```python
from build123d import *

# Parameters (mm, degrees)
M12X1_5_1_D              = 10.5
PATTERN_CIRCULAR_1_COUNT = 8
CHAMFER_1_SIZE           = 8
CHAMFER_2_SIZE           = 2


with BuildPart() as part:
    # 草圖1 → 旋轉1 (revolve)
    with BuildSketch(Plane.XY, mode=Mode.PRIVATE) as revolve_1_sk:
        Polygon((50, 0), (85, 0), (85, 30), (60, 30), (60, 540), (85, 540), (85, 570), (50, 570), align=None)
    revolve(revolve_1_sk.sketch.rotate(Axis((0, -1001.13524313, 0), (0, 1, 0)), 90), axis=Axis((0, -1001.13524313, 0), (0, 1, 0)))

    # 草圖2 → 除料-旋轉1 (revolve, cut)
    with BuildSketch(Plane.XY, mode=Mode.PRIVATE) as cut_revolve_1_sk:
        with BuildLine():
            Line((60, 540), (60, 532))
            ThreePointArc((60, 532), (58, 536), (60, 540))
        make_face()
        with BuildLine():
            Line((60, 38), (60, 30))
            ThreePointArc((60, 30), (58, 34), (60, 38))
        make_face()
    revolve(cut_revolve_1_sk.sketch.rotate(Axis((0, -1001.13524313, 0), (0, -1, 0)), 90), axis=Axis((0, -1001.13524313, 0), (0, -1, 0)), mode=Mode.SUBTRACT)

    # M12x1.5 螺紋孔1 (through all)
    with Locations(Plane.XZ):
        with Locations((-64.671567276, 26.787840266)):
            m12x1_5_1 = Hole(M12X1_5_1_D / 2)

    # 環狀複製排列1: M12x1.5 螺紋孔1 ×8 about axis
    pattern_circular_1_axis = Axis((0, 0, 0), (0, 1, 0))
    for i in range(1, PATTERN_CIRCULAR_1_COUNT):
        add(m12x1_5_1.rotate(pattern_circular_1_axis, i * 360 / PATTERN_CIRCULAR_1_COUNT), mode=Mode.SUBTRACT)

    # 導角1
    chamfer_1_edges = [part.edges().sort_by_distance(p)[0] for p in [
        (0, 540, 85),
        (0, 30, 85),
    ]]
    chamfer(chamfer_1_edges, length=CHAMFER_1_SIZE)

    # 導角2
    chamfer_2_edges = [part.edges().sort_by_distance(p)[0] for p in [
        (0, 570, 85),
        (0, 0, 85),
    ]]
    chamfer(chamfer_2_edges, length=CHAMFER_2_SIZE)


solid = part.part
```
Check sheet for the modelled part. Datum: model origin and axes. Units: mm. A direction names the side the tool comes from. Round coordinates to 2 decimals unless told otherwise and drop trailing zeros. Write each loop counter-clockwise with the first axis right and the second up, starting at its lowest first coordinate (ties: lowest second). Pieces come first, ordered by that corner, then holes. Notation, with made-up numbers: (-6, -29) -> (9, -29) arc R14 ccw to (9, -11) -> close; hole circle Ø5 at (5, 25). An arc over 180 degrees is marked (long way). Put each result on its own line as item: value.
(1) Tool access check on faces 1 (the face through (45, 540, 40)), 2 (the face through (-69.33, 555.21, -29.21)). Record the directions out of +Z, -Z, +X, -X, +Y, -Y that give a thin tool (end or side, any length) a straight path to the whole face; none if there is none.
Values found:
face 1: none
face 2: +Y, -Y
(2) Sectioned sample at B-B (x = 0). Enter the section's corners in (y, z), plus the area to 3 significant figures.
Values found:
outline: (0, -83) -> (2, -85) -> (22, -85) -> (30, -77) -> (30, -60) arc R5 cw to (38, -60) -> (532, -60) arc R5 cw to (540, -60) -> (540, -77) -> (548, -85) -> (568, -85) -> (570, -83) -> (570, -50) -> (0, -50) -> close; (0, 50) -> (570, 50) -> (570, 83) -> (568, 85) -> (548, 85) -> (540, 77) -> (540, 60) arc R5 cw to (532, 60) -> (38, 60) arc R5 cw to (30, 60) -> (30, 77) -> (22, 85) -> (2, 85) -> (0, 83) -> close
area: 14,200 mm^2
(3) Sectioned sample at A-A (z = 0). Enter the section's corners in (x, y).
Values found:
outline: (-85, 2) -> (-83, 0) -> (-50, 0) -> (-50, 570) -> (-83, 570) -> (-85, 568) -> (-85, 548) -> (-77, 540) -> (-60, 540) arc R5 cw to (-60, 532) -> (-60, 38) arc R5 cw to (-60, 30) -> (-77, 30) -> (-85, 22) -> close; (50, 0) -> (83, 0) -> (85, 2) -> (85, 22) -> (77, 30) -> (60, 30) arc R5 cw to (60, 38) -> (60, 532) arc R5 cw to (60, 540) -> (77, 540) -> (85, 548) -> (85, 568) -> (83, 570) -> (50, 570) -> close
(4) Sectioned sample at C-C (y = 277.5). Enter the section's corners in (x, z).
Values found:
outline: circle Ø120 at (0, 0); hole circle Ø100 at (0, 0)
(5) Go/stop test with flat-tipped pins: pin 1 Ø6.5 at (x, z) = (-26.79, 64.67) entering from -Y; pin 2 Ø17 at (x, z) = (64.67, -26.79) entering from -Y; pin 3 Ø3 at (x, y) = (43.5, 358) entering from -Z; pin 4 Ø2 at (y, z) = (258.5, -7) entering from -X. Record where each tip stops, or that it passes through.
Values found:
pin 1: passes through
pin 2: stops at y = 0
pin 3: stops at z = -42.85
pin 4: stops at x = -59.7
(6) Mould release check, pull along Y, two halves, no side actions. Record for faces 3 (the face through (45, 30, -40)), 4 (the face through (81.148, 569.875, 18.02)), 5 (the face through (69.33, 555.21, 29.21)): released by +Y, released by -Y, zero draft, split by the parting line, or undercut.
Values found:
face 3: undercut
face 4: released by +Y
face 5: zero draft
(7) Material ranges on line 1 (Y direction, x = 26.5, z = 58); line 2 (X direction, y = 525.5, z = -3); line 3 (Z direction, x = -11, y = 434) (3 decimals), recorded low to high.
Values found:
line 1: y = 0 to 30, 540 to 570
line 2: x = -59.92 to -49.91, 49.91 to 59.92
line 3: z = -58.983 to -48.775, 48.775 to 58.983
